```python
from build123d import *

# Parameters (mm, degrees)
SKETCH_1_R      = 1.4
EXTRUDE_1_DEPTH = 37.55


with BuildPart() as part:
    # 草图1 → 凸台-拉伸1 (new body)
    with BuildSketch(Plane(origin=(0, 0, 0), x_dir=(1, 0, 0), z_dir=(0, 1, 0))):
        with BuildLine():
            Line((4.448985647, -10.849582747), (4.448985647, 9.150417253))
            Line((4.448985647, 9.150417253), (24.448985647, 9.150417253))
            ThreePointArc((24.448985647, 9.150417253), (29.448985647, 14.150417253), (24.448985647, 19.150417253))
            Line((24.448985647, 19.150417253), (-35.551014353, 19.150417253))
            ThreePointArc((-35.551014353, 19.150417253), (-40.551014353, 14.150417253), (-35.551014353, 9.150417253))
            Line((-35.551014353, 9.150417253), (-15.551014353, 9.150417253))
            Line((-15.551014353, 9.150417253), (-15.551014353, -10.849582747))
            Line((-15.551014353, -10.849582747), (-35.551014353, -10.849582747))
            ThreePointArc((-35.551014353, -10.849582747), (-40.551014353, -15.849582747), (-35.551014353, -20.849582747))
            Line((-35.551014353, -20.849582747), (24.448985647, -20.849582747))
            ThreePointArc((24.448985647, -20.849582747), (29.448985647, -15.849582747), (24.448985647, -10.849582747))
            Line((24.448985647, -10.849582747), (4.448985647, -10.849582747))
        make_face()
        with Locations(Location((24.448985647, 14.150417253, 0), (0, 0, 270))):
            Circle(SKETCH_1_R, mode=Mode.SUBTRACT)
        with Locations(Location((24.448985647, -15.849582747, 0), (0, 0, 90))):
            Circle(SKETCH_1_R, mode=Mode.SUBTRACT)
        with Locations(Location((-5.551014353, 14.150417253, 0), (0, 0, 270))):
            Circle(SKETCH_1_R, mode=Mode.SUBTRACT)
        with Locations(Location((-5.551014353, -0.849582747, 0), (0, 0, 270))):
            Circle(SKETCH_1_R, mode=Mode.SUBTRACT)
        with Locations(Location((-5.551014353, -15.849582747, 0), (0, 0, 90))):
            Circle(SKETCH_1_R, mode=Mode.SUBTRACT)
        with Locations(Location((-35.551014353, -15.849582747, 0), (0, 0, 270))):
            Circle(SKETCH_1_R, mode=Mode.SUBTRACT)
        with Locations(Location((-35.551014353, 14.150417253, 0), (0, 0, 90))):
            Circle(SKETCH_1_R, mode=Mode.SUBTRACT)
    extrude(amount=EXTRUDE_1_DEPTH)


solid = part.part
```
CAD build for the part. Positions are in the model's coordinates, mm. A direction names the side the tool comes from. Round coordinates to 2 decimals unless told otherwise and drop trailing zeros. Write each loop counter-clockwise with the first axis right and the second up, starting at its lowest first coordinate (ties: lowest second). Pieces come first, ordered by that corner, then holes. Notation, with made-up numbers: M 36,46 L 93,46 A19 cw 93,62 Z; hole C 14.5,-31.75 d4. An arc over 180 degrees is marked long. One line per question, with ' | ' between items.
1. Probe L1, parallel to Z at x = 24.5, y = 2; L2, parallel to Z at x = 16, y = 5.5; L3, parallel to X at y = 18, z = 16.5. List the from-to ranges inside material, lowest first. Write a range as from..to.
Working result:
L1: -19.15..-15.55, -12.75..-9.15, 10.85..14.45, 17.25..20.85 | L2: -19.15..-9.15, 10.85..20.85 | L3: -40.51..-36.79, -34.31..-6.79, -4.31..23.21, 25.69..29.41
2. Cut at A-A on x = -23. Write the cut outline in (y, z).
Working result:
outline: M 0,-19.15 L 37.55,-19.15 L 37.55,-9.15 L 0,-9.15 Z; M 0,10.85 L 37.55,10.85 L 37.55,20.85 L 0,20.85 Z
3. Pin check, flat tips, straight feed: pin 1 Ø3 at (x, z) = (-5.55, 15.85) entering from +Y; pin 2 Ø6 at (y, z) = (16.5, -4) entering from +X; pin 3 Ø12 at (y, z) = (14.5, 8.5) entering from -X; pin 4 Ø22 at (y, z) = (19, 0) entering from -X. Stop position of each tip, or through.
Working result:
pin 1: y = 37.55 | pin 2: x = 4.45 | pin 3: x = -40.37 | pin 4: x = -39.43
4. Mould opens along Z. For faces 4 (the flat face through (-6, 19, 20.85)), 5 (the flat face through (-5, 19, -19.15)), 6 (the flat face through (-25, 19, 10.85)) say: pulls with the +Z half, pulls with the -Z half, needs draft (parallel to the pull), parting line crosses it, or undercut.
Working result:
face 4: pulls with the +Z half | face 5: pulls with the -Z half | face 6: undercut
5. Cut at B-B on y = 14. Write the cut outline in (x, z).
Working result:
outline: M -35.55,-19.15 L 24.45,-19.15 A5 ccw 24.45,-9.15 L 4.45,-9.15 L 4.45,10.85 L 24.45,10.85 A5 ccw 24.45,20.85 L -35.55,20.85 A5 ccw -35.55,10.85 L -15.55,10.85 L -15.55,-9.15 L -35.55,-9.15 A5 ccw Z; hole C -35.55,-14.15 d2.8; hole C -35.55,15.85 d2.8; hole C -5.55,-14.15 d2.8; hole C -5.55,0.85 d2.8; hole C -5.55,15.85 d2.8; hole C 24.45,-14.15 d2.8; hole C 24.45,15.85 d2.8
6. Cut at D-D on z = -17. Write the cut outline in (x, y).
Working result:
outline: M -39.66,0 L 28.56,0 L 28.56,37.55 L -39.66,37.55 Z
7. Which spindle directions (+Z, -Z, +X, -X, +Y, -Y) get a long thin tool onto all of the face, cutting with end or side? Do faces 1 (the flat face through (-26, 19, -9.15)), 2 (the cylindrical face through (-34.163, 18.512, 15.667)), 3 (the flat face through (4.449, 19, 1)). Say none if no direction does.
Working result:
face 1: -X, +Y, -Y | face 2: +Y, -Y | face 3: +X, +Y, -Y
8. Cut at C-C on z = -6.5. Write the cut outline in (x, y).
Working result:
outline: M -15.55,0 L 4.45,0 L 4.45,37.55 L -15.55,37.55 Z
